```python
from build123d import *

# Parameters (mm, degrees)
SKETCH1_R           = 4.7625
SKETCH1_R_2         = 2.5
BOSS_EXTRUDE1_DEPTH = 3.96875
SKETCH2_R           = 9
SKETCH2_R_2         = 2.5
BOSS_EXTRUDE2_DEPTH = 9
SKETCH3_W           = 3
SKETCH3_H           = 8


with BuildPart() as part:
    # Sketch1 → Boss-Extrude1 (new, symmetric)
    with BuildSketch(Plane(origin=(0, 0, 0), x_dir=(1, 0, 0), z_dir=(0, 1, 0))):
        with Locations(Location((0, 0, 0), (0, 0, 270))):
            Circle(SKETCH1_R)
        with Locations(Location((0, 0, 0), (0, 0, 270))):
            Circle(SKETCH1_R_2, mode=Mode.SUBTRACT)
    extrude(amount=BOSS_EXTRUDE1_DEPTH, both=True)

    # Sketch2 → Boss-Extrude2 (add)
    with BuildSketch(Plane(origin=(0, 3.96875, 0), x_dir=(1, 0, 0), z_dir=(0, 1, 0))):
        with Locations(Location((0, 0, 0), (0, 0, 270))):
            Circle(SKETCH2_R)
        with Locations(Location((0, 0, 0), (0, 0, 270))):
            Circle(SKETCH2_R_2, mode=Mode.SUBTRACT)
    extrude(amount=BOSS_EXTRUDE2_DEPTH)

    # Sketch3 → Cut-Revolve1 (revolve, cut)
    with BuildSketch(Plane(origin=(0, 0, 0), x_dir=(0, 0, -1), z_dir=(1, 0, 0)), mode=Mode.PRIVATE) as cut_revolve1_sk:
        with Locations((7.5, 8.46875)):
            Rectangle(SKETCH3_W, SKETCH3_H)
    revolve(cut_revolve1_sk.sketch.rotate(Axis((0, 3.96875, 0), (0, -1, 0)), 180), axis=Axis((0, 3.96875, 0), (0, -1, 0)), mode=Mode.SUBTRACT)


solid = part.part
```
The model under review builds one solid part; all positions refer to its coordinate system, in mm. A direction names the side the tool comes from. Round coordinates to 2 decimals unless told otherwise and drop trailing zeros. Write each loop counter-clockwise with the first axis right and the second up, starting at its lowest first coordinate (ties: lowest second). Pieces come first, ordered by that corner, then holes. Notation, with made-up numbers: M 81,-32 L 99,-32 A23 cw 99,-9 Z; hole C -1.75,39 d2. An arc over 180 degrees is marked long. Use CSV: the item, a comma, the result in double quotes. Start each with the question number.
(1) The part is to be moulded in two halves that separate along Y. For faces 1 (the face through (-2, -3.969, 2)), 2 (the face through (-2.9, 0.06, -3.78)), 3 (the face through (6, 12.469, -2)), say which applies: +Y half, -Y half, draft (parallel to the pull), parting line (faces both ways), or undercut.
(2) We need section D-D, the plane z = -4.5. State the section outline as (x, y) points.
(3) For line 1 along X through (y, z) = (5.5, 0); line 2 along Y through (x, z) = (-4.75, -6.5); line 3 along X through (y, z) = (0, 0), list the stretches that pass through material, from the lowest coordinate up.
(4) We need section B-B, the plane z = 0. State the section outline as (x, y) points.
(5) We need section C-C, the plane y = 2.5. State the section outline as (x, z) points (1 decimal), then the cut area to 3 significant figures.
(6) Clearance check with flat-ended pins moving along their axes: P1, Ø10, axis at y = 4.5, z = -0.5, coming from the -X side; P2, Ø2, axis at x = 1, y = 9.5, coming from the +Z side; P3, Ø4, axis at x = -7, z = -5, coming from the -Y side; P4, Ø1.5, axis at x = 5, y = 4, coming from the +Z side. State where each tip first meets the part, or that it passes through.
(7) Tool access review of faces 4 (the face through (-1.802, 8.525, 5.723)), 5 (the face through (-2.44, 4.38, -0.54)), 6 (the face through (-4, 3.969, 4)): name each direction out of +Z, -Z, +X, -X, +Y, -Y from which nothing blocks a thin tool from reaching the whole face with its end or side.
(8) We need section A-A, the plane x = 0. State the section outline as (y, z) points.
Findings:
1,face 1,"-Y half"
1,face 2,"draft"
1,face 3,"undercut"
2,outline,"M -7.79,3.97 L -1.56,3.97 L -1.56,-3.97 L 1.56,-3.97 L 1.56,3.97 L 7.79,3.97 L 7.79,4.47 L 3.97,4.47 L 3.97,12.47 L 7.79,12.47 L 7.79,12.97 L -7.79,12.97 L -7.79,12.47 L -3.97,12.47 L -3.97,4.47 L -7.79,4.47 Z"
3,line 1,"-6 to -2.5, 2.5 to 6"
3,line 2,"3.97 to 4.47, 12.47 to 12.97"
3,line 3,"-4.76 to -2.5, 2.5 to 4.76"
4,outline,"M -9,3.97 L -4.76,3.97 L -4.76,-3.97 L -2.5,-3.97 L -2.5,12.97 L -9,12.97 L -9,12.47 L -6,12.47 L -6,4.47 L -9,4.47 Z; M 2.5,-3.97 L 4.76,-3.97 L 4.76,3.97 L 9,3.97 L 9,4.47 L 6,4.47 L 6,12.47 L 9,12.47 L 9,12.97 L 2.5,12.97 Z"
5,outline,"C 0,0 d9.5; hole C 0,0 d5"
5,area,"51.6 mm^2"
6,P1,"x = -9"
6,P2,"z = 6"
6,P3,"y = 3.97"
6,P4,"z = 7.93"
7,face 4,"none"
7,face 5,"+Y, -Y"
7,face 6,"-Y"
8,outline,"M -3.97,-4.76 L 3.97,-4.76 L 3.97,-9 L 4.47,-9 L 4.47,-6 L 12.47,-6 L 12.47,-9 L 12.97,-9 L 12.97,-2.5 L -3.97,-2.5 Z; M -3.97,2.5 L 12.97,2.5 L 12.97,9 L 12.47,9 L 12.47,6 L 4.47,6 L 4.47,9 L 3.97,9 L 3.97,4.76 L -3.97,4.76 Z"
